The listing builds one solid part. Answer for the finished solid, in the listing's coordinates (mm). A direction names the side the tool comes from. Give positions to 0.01 mm unless a question says otherwise; leave off trailing zeros. Order: outer loops, then holes, each group sorted by start corner. A loop starts at its lowest first (then second) coordinate and runs counter-clockwise, first axis right, second up. Notation, with made-up numbers: (58, 9.25) - (95, 9.25) arc R24 ccw to (95, 29.25) - close; hole circle Ø7 at (-11, 43.5). An arc over 180 degrees is marked (long way). Answer as CSV lines item,"result". Start each with the question number.
1. Section D-D on z = 14.5 is taken. Give the vertices of the cut face in (x, y), and give its area (3 significant figures).
2. Which of the six approach directions +Z, -Z, +X, -X, +Y, -Y give full straight-line access (tool end or side, diameter ignored) to faces 1 (the flat face through (-19, 30, 22.5)), 2 (the flat face through (1, 1, 0)), 3 (the cylindrical face through (-34.576, 10.889, 20.218))?
3. Flat-ended cylindrical pins translate along their axes: pin 1 (3 mm diameter, centred on x = 6, z = 6.5, fed in from +Y); pin 2 (1 mm diameter, centred on x = -32.5, z = 11, fed in from -Y); pin 3 (1.5 mm diameter, centred on y = 13, z = 25, fed in from +X). Find the tip coordinate at first contact, or state that the pin passes through.
4. Section A-A on y = 0 is taken. Give the vertices of the cut face in (x, z), and give its area (3 significant figures).
5. Section C-C on z = 21.5 is taken. Give the vertices of the cut face in (x, y).
6. Consider line 1 along X through (y, z) = (-15.5, 9.25); line 2 along X through (y, z) = (-10.5, 15); line 3 along Y through (x, z) = (8.5, 20). Determine where each line is inside the solid, lowest interval first. Write a range as [from, to].
7. Determine the mould class of faces 4 (the cylindrical face through (-39.584, 12.465, 11.409)), 5 (the flat face through (19, 30, 26)), 6 (the cylindrical face through (25.76, 23.62, 24.23)), 7 (the flat face through (0, 0, 29)) for opening direction Z: +Z half, -Z half, draft (parallel to the pull), parting line (faces both ways), or undercut.
from build123d import *

# Parameters (mm, degrees)
F2_R = 5
F3_R = 2


with BuildPart() as f1:
    # F0 (on Front) → F1 (revolve)
    with BuildSketch(Plane.XZ):
        Polygon((-36.25, 22.5), (-36.25, 18), (-41.5, 18), (-41.5, 0), (0, 0), (0, 18), (0, 29), (-36.25, 29), (-36.25, 26), (-34.95, 26), (-34.95, 22.5), align=None)
    revolve(axis=Axis((0, 0, 9), (0, 0, -1)))

    # F2
    f2_edges = [f1.edges().sort_by_distance(p)[0] for p in [
        (41.5, 0, 0),
    ]]
    fillet(f2_edges, radius=F2_R)

    # F3
    f3_edges = [f1.edges().sort_by_distance(p)[0] for p in [
        (36.25, 0, 29),
    ]]
    fillet(f3_edges, radius=F3_R)


solid = f1.part
Checks:
1,outline,"circle Ø83 at (0, 0)"
1,area,"5,410 mm²"
2,face 1,"none"
2,face 2,"-Z, +X, -X, +Y, -Y"
2,face 3,"+Z"
3,pin 1,"stops at y = 41.26"
3,pin 2,"stops at y = -26.42"
3,pin 3,"stops at x = 32.73"
4,outline,"(-41.5, 5) arc R5 ccw to (-36.5, 0) - (36.5, 0) arc R5 ccw to (41.5, 5) - (41.5, 18) - (36.25, 18) - (36.25, 22.5) - (34.95, 22.5) - (34.95, 26) - (36.25, 26) - (36.25, 27) arc R2 ccw to (34.25, 29) - (-34.25, 29) arc R2 ccw to (-36.25, 27) - (-36.25, 26) - (-34.95, 26) - (-34.95, 22.5) - (-36.25, 22.5) - (-36.25, 18) - (-41.5, 18) - close"
4,area,"2,270 mm²"
5,outline,"circle Ø72.5 at (0, 0)"
6,line 1,"x = [-38.5, 38.5]"
6,line 2,"x = [-40.15, 40.15]"
6,line 3,"y = [-35.24, 35.24]"
7,face 4,"draft"
7,face 5,"undercut"
7,face 6,"undercut"
7,face 7,"+Z half"
